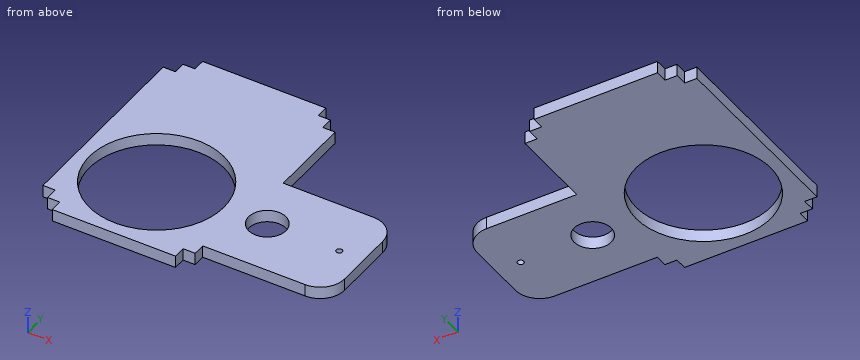
```python
from build123d import *

# Parameters (mm, degrees)
SKETCH1_R           = 35.1155
SKETCH1_R_2         = 9.7234375
SKETCH1_R_3         = 1.5875
BOSS_EXTRUDE1_DEPTH = 6.35


with BuildPart() as part:
    # Sketch1 → Boss-Extrude1 (new body)
    with BuildSketch(Plane.XY):
        with BuildLine():
            Line((-35.1155, -35.1155), (-28.7655, -35.1155))
            Line((-28.7655, -35.1155), (-28.7655, -41.4655))
            Line((-28.7655, -41.4655), (35.5219, -41.4655))
            Line((35.5219, -41.4655), (35.5219, -35.1155))
            Line((35.5219, -35.1155), (41.8719, -35.1155))
            Line((41.8719, -35.1155), (41.8719, -28.7655))
            Line((41.8719, -28.7655), (95.3008, -28.7655))
            ThreePointArc((95.3008, -28.7655), (104.281056121, -25.045756121), (108.0008, -16.0655))
            Line((108.0008, -16.0655), (108.0008, 16.0655))
            ThreePointArc((108.0008, 16.0655), (104.281056121, 25.045756121), (95.3008, 28.7655))
            Line((95.3008, 28.7655), (48.2219, 28.7655))
            Line((48.2219, 28.7655), (48.2219, 72.4027))
            Line((48.2219, 72.4027), (41.8719, 72.4027))
            Line((41.8719, 72.4027), (41.8719, 78.7527))
            Line((41.8719, 78.7527), (35.5219, 78.7527))
            Line((35.5219, 78.7527), (35.5219, 85.1027))
            Line((35.5219, 85.1027), (-28.7655, 85.1027))
            Line((-28.7655, 85.1027), (-28.7655, 78.7527))
            Line((-28.7655, 78.7527), (-35.1155, 78.7527))
            Line((-35.1155, 78.7527), (-35.1155, 72.4027))
            Line((-35.1155, 72.4027), (-41.4655, 72.4027))
            Line((-41.4655, 72.4027), (-41.4655, -28.7655))
            Line((-41.4655, -28.7655), (-35.1155, -28.7655))
            Line((-35.1155, -28.7655), (-35.1155, -35.1155))
        make_face()
        Circle(SKETCH1_R, mode=Mode.SUBTRACT)
        with Locations((57.7469, 0)):
            Circle(SKETCH1_R_2, mode=Mode.SUBTRACT)
        with Locations((95.3008, 0)):
            Circle(SKETCH1_R_3, mode=Mode.SUBTRACT)
    extrude(amount=-BOSS_EXTRUDE1_DEPTH)


solid = part.part
```
Here's how the part is built. I have some questions about the finished solid (model axes, mm). Round coordinates to 2 decimals unless told otherwise and drop trailing zeros. Write each loop counter-clockwise with the first axis right and the second up, starting at its lowest first coordinate (ties: lowest second). Pieces come first, ordered by that corner, then holes.
Q1. If we section it at A-A on y = 0: Write out the boundary of the cut face in (x, z).
Q2. If we section it at D-D on y = -21.5: Write out the boundary of the cut face in (x, z), plus the area to 3 significant figures.
Q3. If we section it at C-C on z = -4.25: Write out the boundary of the cut face in (x, y) (1 decimal).
Q4. If we section it at B-B on x = 0: Write out the boundary of the cut face in (y, z).
Q5. Will these pins go through, and if not, where does the flat tip stop? P1, Ø1, axis at x = 90, z = -4.5, coming from the -Y side; P2, Ø3, axis at y = 83, z = -3.5, coming from the -X side; P3, Ø1.9, axis at y = 75, z = -2, coming from the -X side; P4, Ø15.5, axis at x = 57.75, y = 0, coming from the -Z side.
Q6. Please list where these lines run through material, in increasing order: probe 1 along Y at (x, z) = (95, -2); probe 2 along Y at (x, z) = (0, -4.5); probe 3 along Y at (x, z) = (44, -1.5).
Answer below:
1. outline: (-41.47, -6.35) - (-35.12, -6.35) - (-35.12, 0) - (-41.47, 0) - close; (35.12, -6.35) - (48.02, -6.35) - (48.02, 0) - (35.12, 0) - close; (67.47, -6.35) - (93.71, -6.35) - (93.71, 0) - (67.47, 0) - close; (96.89, -6.35) - (108, -6.35) - (108, 0) - (96.89, 0) - close
2. outline: (-41.47, -6.35) - (-27.76, -6.35) - (-27.76, 0) - (-41.47, 0) - close; (27.76, -6.35) - (106.78, -6.35) - (106.78, 0) - (27.76, 0) - close
2. area: 589 mm2
3. outline: (-41.5, -28.8) - (-35.1, -28.8) - (-35.1, -35.1) - (-28.8, -35.1) - (-28.8, -41.5) - (35.5, -41.5) - (35.5, -35.1) - (41.9, -35.1) - (41.9, -28.8) - (95.3, -28.8) arc R12.7 ccw to (108, -16.1) - (108, 16.1) arc R12.7 ccw to (95.3, 28.8) - (48.2, 28.8) - (48.2, 72.4) - (41.9, 72.4) - (41.9, 78.8) - (35.5, 78.8) - (35.5, 85.1) - (-28.8, 85.1) - (-28.8, 78.8) - (-35.1, 78.8) - (-35.1, 72.4) - (-41.5, 72.4) - close; hole circle Ø70.2 at (0, 0); hole circle Ø19.4 at (57.7, 0); hole circle Ø3.2 at (95.3, 0)
4. outline: (-41.47, -6.35) - (-35.12, -6.35) - (-35.12, 0) - (-41.47, 0) - close; (35.12, -6.35) - (85.1, -6.35) - (85.1, 0) - (35.12, 0) - close
5. P1: stops at y = -28.77
5. P2: stops at x = -28.77
5. P3: stops at x = -35.12
5. P4: passes through
6. probe 1: y = -28.77 to -1.56, 1.56 to 28.77
6. probe 2: y = -41.47 to -35.12, 35.12 to 85.1
6. probe 3: y = -28.77 to 72.4
